Can you work these out from the drawing? Everything is in mm from the part's minimum corner. A direction names the side the tool comes from. Round coordinates to 2 decimals unless told otherwise and drop trailing zeros. Order: outer loops, then holes, each group sorted by start corner. A loop starts at its lowest first (then second) coordinate and runs counter-clockwise, first axis right, second up. Notation, with made-up numbers: (87.5, 6) -> (96.5, 6) arc R14 ccw to (96.5, 21) -> close; hole circle Ø7 at (20, 4.25). An arc over 180 degrees is marked (long way). One line per item, written item: value.
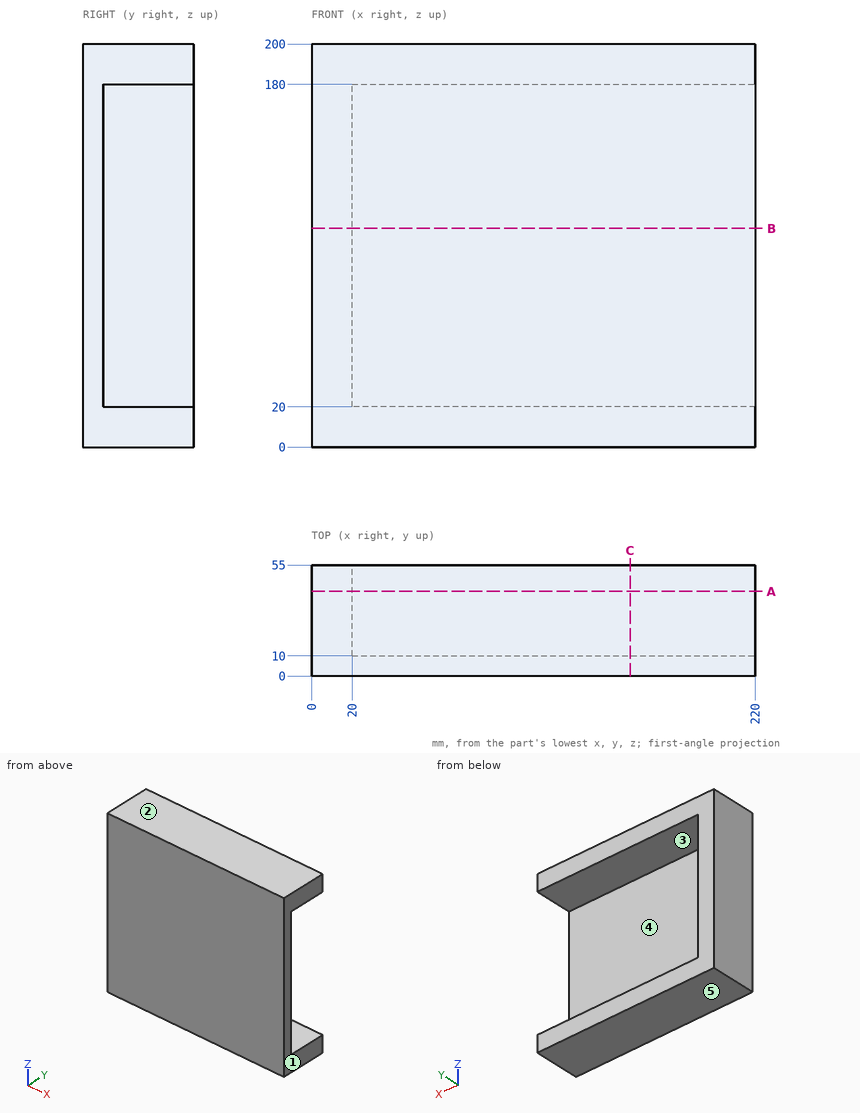
Q1. I want a section at B-B on z = 108.5. List the corners of the cut face in (x, y) for me, plus the area to 3 significant figures.
Answers below:
outline: (0, 0) -> (220, 0) -> (220, 10) -> (20, 10) -> (20, 55) -> (0, 55) -> close
area: 3,100 mm^2
Q2. We'd pull the mould along Z, two halves only. Please class the marked faces 1, 2 and 3: released by +Z, released by -Z, zero draft, split by the parting line, or undercut.
Answers below:
face 1: zero draft
face 2: released by +Z
face 3: undercut
Q3. Please list where these lines run through material, in increasing order: line 1 along Z through (x, y) = (199.5, 13); line 2 along X through (y, z) = (27, 45.5); line 3 along Y through (x, z) = (141, 59).
Answers below:
line 1: 0 to 20, 180 to 200
line 2: 0 to 20
line 3: 0 to 10
Q4. I want a section at C-C on x = 158. List the corners of the cut face in (y, z) for me, plus the area to 3 significant figures.
Answers below:
outline: (0, 0) -> (55, 0) -> (55, 20) -> (10, 20) -> (10, 180) -> (55, 180) -> (55, 200) -> (0, 200) -> close
area: 3,800 mm^2
Q5. I want a section at A-A on y = 42. List the corners of the cut face in (x, z) for me.
Answers below:
outline: (0, 0) -> (220, 0) -> (220, 20) -> (20, 20) -> (20, 180) -> (220, 180) -> (220, 200) -> (0, 200) -> close
Q6. On a 3-axis mill with a long thin cutter (end or side, diameter ignored), from which of +Z, -Z, +X, -X, +Y, -Y can I reach the whole of each face in a straight line? I mean the marked faces 4 and 5. Say none if no direction works.
Answers below:
face 4: +X, +Y
face 5: -Z, +X, -X, +Y, -Y
Q7. Will these pins go through, and if not, where does the flat tip stop? pin 1 Ø22.5 at (y, z) = (24.5, 62) entering from +X; pin 2 Ø2 at (x, z) = (94.5, 32.5) entering from +Y.
Answers below:
pin 1: x = 20
pin 2: y = 10
